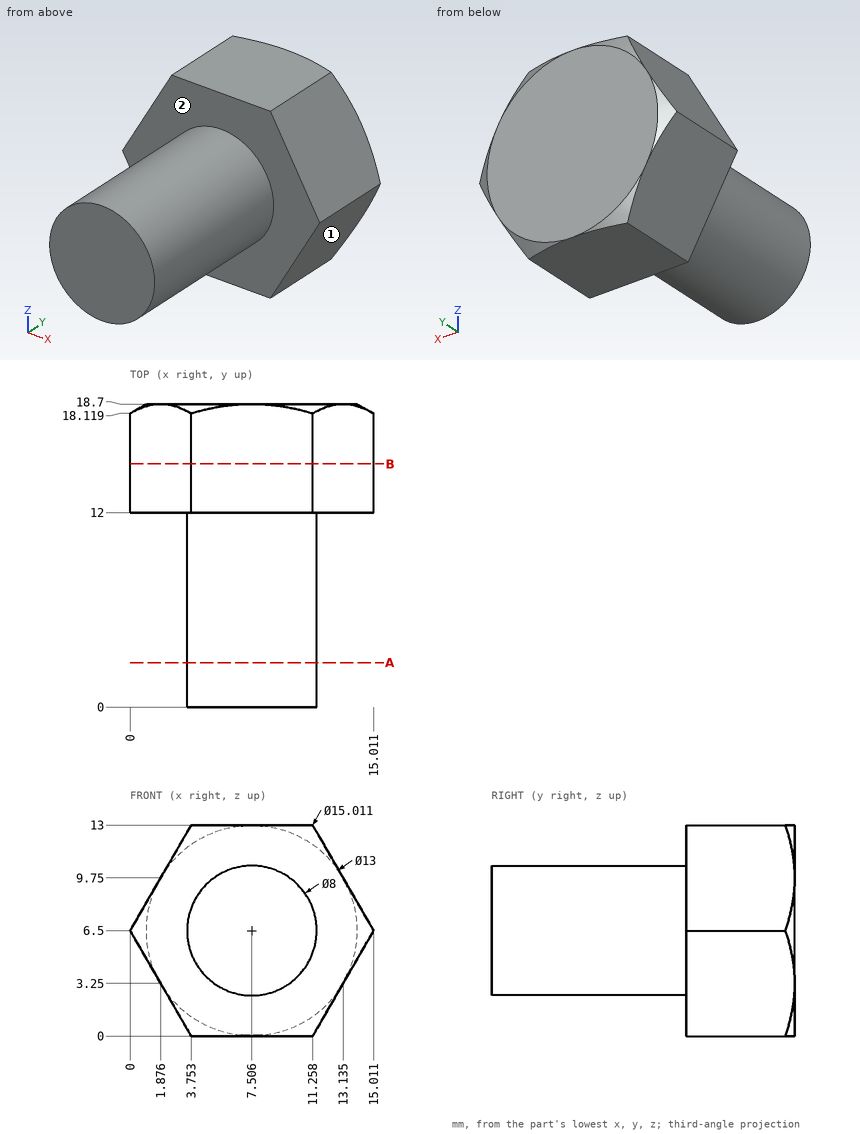
Answer from the drawing. Dimensions are ordinates in mm from the lowest x, y and z of the part. A direction names the side the tool comes from. Give positions to 0.01 mm unless a question says otherwise; leave off trailing zeros. Order: outer loops, then holes, each group sorted by start corner. A loop starts at its lowest first (then second) coordinate and runs counter-clockwise, first axis right, second up.
(1) Straight lines are drawn through the part: L1, parallel to Y at x = 11.75, z = 8.5; L2, parallel to X at y = 1.25, z = 9 (1 decimal); L3, parallel to X at y = 10.75, z = 10 (1 decimal). For each, find the intervals that lie inside material, in ascending order.
(2) Find section B-B (y = 15). Give the vertices of the cut face in (x, z), plus the area to 3 significant figures.
(3) Find section A-A (y = 2.75). Give the vertices of the cut face in (x, z) (1 decimal).
(4) Given pin 1 (1.5 mm diameter, centred on x = 11, y = 8, fed in from +Z); pin 2 (6 mm diameter, centred on y = 4.5, z = 6.5, fed in from -X); pin 3 (3 mm diameter, centred on y = 11.5, z = 9.5, fed in from -X) (1 decimal), each flat-ended and moving along its own axis, determine where each tip first touches the part or whether it passes through.
(5) For the marked faces 1 and 2, determine the directions among +Z, -Z, +X, -X, +Y, -Y from which every point of the face is accessible in a straight line to the end or side of a thin tool.
Result sheet:
1. L1: y = 12 to 18.7
1. L2: x = 4.4 to 10.6
1. L3: x = 5.6 to 9.4
2. outline: (0, 6.5) - (3.75, 0) - (11.26, 0) - (15.01, 6.5) - (11.26, 13) - (3.75, 13) - close
2. area: 146 mm2
3. outline: circle Ø8 at (7.5, 6.5)
4. pin 1: stops at z = 9.41
4. pin 2: stops at x = 3.51
4. pin 3: stops at x = 0.9
5. face 1: -Z, +X, +Y, -Y
5. face 2: -Y
